from build123d import *

# Parameters (mm, degrees)
F0_R     = 1.55
F0_R_2   = 3
F1_DEPTH = 5
F2_DEPTH = 8


with BuildPart() as f1:
    # F0 (on Top) → F1 (new body)
    with BuildSketch(Plane.XY):
        with BuildLine():
            ThreePointArc((9.1651513899, -4), (9.7890631293, -2.0430964369), (10, 0))
            ThreePointArc((10, 0), (9.7890631293, 2.0430964369), (9.1651513899, 4))
            ThreePointArc((9.1651513899, 4), (5.4772255751, 8.3666002653), (0, 10))
            ThreePointArc((0, 10), (-10, 0), (0, -10))
            ThreePointArc((0, -10), (5.4772255751, -8.3666002653), (9.1651513899, -4))
        make_face()
        with Locations((0, -6.35)):
            Circle(F0_R, mode=Mode.SUBTRACT)
        with Locations((-6.35, 0)):
            Circle(F0_R, mode=Mode.SUBTRACT)
        Circle(F0_R_2, mode=Mode.SUBTRACT)
        with Locations((6.35, 0)):
            Circle(F0_R, mode=Mode.SUBTRACT)
        with Locations((0, 6.35)):
            Circle(F0_R, mode=Mode.SUBTRACT)
        with BuildLine():
            ThreePointArc((0, 10), (5.4772255751, 8.3666002653), (9.1651513899, 4))
            Line((9.1651513899, 4), (90.8348486101, 4))
            ThreePointArc((90.8348486101, 4), (94.5227744249, 8.3666002653), (100, 10))
            Line((100, 10), (0, 10))
        make_face()
        with BuildLine():
            ThreePointArc((100, 10), (94.5227744249, 8.3666002653), (90.8348486101, 4))
            Line((90.8348486101, 4), (100, 4))
            ThreePointArc((100, 4), (102.8284271247, 2.8284271247), (104, 0))
            ThreePointArc((104, 0), (102.8284271247, -2.8284271247), (100, -4))
            Line((100, -4), (90.8348486101, -4))
            ThreePointArc((90.8348486101, -4), (94.5227744249, -8.3666002653), (100, -10))
            ThreePointArc((100, -10), (107.0710678119, -7.0710678119), (110, 0))
            ThreePointArc((110, 0), (107.0710678119, 7.0710678119), (100, 10))
        make_face()
        with BuildLine():
            Line((90.8348486101, -4), (9.1651513899, -4))
            ThreePointArc((9.1651513899, -4), (5.4772255751, -8.3666002653), (0, -10))
            Line((0, -10), (100, -10))
            ThreePointArc((100, -10), (94.5227744249, -8.3666002653), (90.8348486101, -4))
        make_face()
        with BuildLine():
            ThreePointArc((9.1651513899, 4), (9.7890631293, 2.0430964369), (10, 0))
            ThreePointArc((10, 0), (9.7890631293, -2.0430964369), (9.1651513899, -4))
            Line((9.1651513899, -4), (90.8348486101, -4))
            ThreePointArc((90.8348486101, -4), (90, 0), (90.8348486101, 4))
            Line((90.8348486101, 4), (9.1651513899, 4))
        make_face()
        with BuildLine():
            Line((100, 4), (90.8348486101, 4))
            ThreePointArc((90.8348486101, 4), (90, 0), (90.8348486101, -4))
            Line((90.8348486101, -4), (100, -4))
            ThreePointArc((100, -4), (96, 0), (100, 4))
        make_face()
    extrude(amount=F1_DEPTH)

    # F0 (on Top) → F2 (join)
    with BuildSketch(Plane.XY):
        with BuildLine():
            ThreePointArc((9.1651513899, -4), (9.7890631293, -2.0430964369), (10, 0))
            ThreePointArc((10, 0), (9.7890631293, 2.0430964369), (9.1651513899, 4))
            ThreePointArc((9.1651513899, 4), (5.4772255751, 8.3666002653), (0, 10))
            ThreePointArc((0, 10), (-10, 0), (0, -10))
            ThreePointArc((0, -10), (5.4772255751, -8.3666002653), (9.1651513899, -4))
        make_face()
        with Locations((0, -6.35)):
            Circle(F0_R, mode=Mode.SUBTRACT)
        with Locations((-6.35, 0)):
            Circle(F0_R, mode=Mode.SUBTRACT)
        Circle(F0_R_2, mode=Mode.SUBTRACT)
        with Locations((6.35, 0)):
            Circle(F0_R, mode=Mode.SUBTRACT)
        with Locations((0, 6.35)):
            Circle(F0_R, mode=Mode.SUBTRACT)
    extrude(amount=F2_DEPTH)


solid = f1.part
The listing builds one solid part. Answer for the finished solid, in the listing's coordinates (mm). Coordinates: 2 decimals unless noted, no trailing zeros. Loops run counter-clockwise (first coordinate to the right, second up) from the corner with the lowest first, then second, coordinate; pieces in that order, holes last. Notation, with made-up numbers: M 54,-10 L 60,-10 A11 cw 60,3 Z; hole C 11.5,82.25 d1. An arc over 180 degrees is marked long. Answer in a Markdown table with one row per item.
1) Find the intervals of material crossed by probe 1 along X at (y, z) = (-2, 1.75); probe 2 along Y at (x, z) = (100, 3); probe 3 along Z at (x, y) = (66, 1.25), in increasing order.
Answers below:
| item | result |
|---|---|
| probe 1 | -9.8 to -2.24, 2.24 to 96.54, 103.46 to 109.8 |
| probe 2 | -10 to -4, 4 to 10 |
| probe 3 | 0 to 5 |
2) Find section D-D (x = -6.35). Determine the outline of the cut face in (y, z).
Answers below:
| item | result |
|---|---|
| outline | M -7.73,0 L -1.55,0 L -1.55,8 L -7.73,8 Z; M 1.55,0 L 7.73,0 L 7.73,8 L 1.55,8 Z |
3) Determine the mould class of faces 1 (the cylindrical face through (-9.76, 2.17, 4.83)), 2 (the flat face through (54, 0, 5)), 3 (the cylindrical face through (0.715, 4.975, 3.944)) for opening direction X: released by +X, released by -X, zero draft, split by the parting line, or undercut.
Answers below:
| item | result |
|---|---|
| face 1 | split by the parting line |
| face 2 | zero draft |
| face 3 | undercut |
4) Find section C-C (x = 6.35). Determine the outline of the cut face in (y, z), then the cut area to 3 significant figures.
Answers below:
| item | result |
|---|---|
| outline | M -10,0 L -1.55,0 L -1.55,8 L -7.73,8 L -7.73,5 L -10,5 Z; M 1.55,0 L 10,0 L 10,5 L 7.73,5 L 7.73,8 L 1.55,8 Z |
| area | 122 mm^2 |
5) Find section B-B (y = -6.35). Determine the outline of the cut face in (x, z), then the cut area to 3 significant figures.
Answers below:
| item | result |
|---|---|
| outline | M -7.73,0 L -1.55,0 L -1.55,8 L -7.73,8 Z; M 1.55,0 L 107.73,0 L 107.73,5 L 7.73,5 L 7.73,8 L 1.55,8 Z |
| area | 599 mm^2 |
6) Find section A-A (z = 2.25). Determine the outline of the cut face in (x, y).
Answers below:
| item | result |
|---|---|
| outline | M 0,-10 L 100,-10 A10 ccw 100,10 L 0,10 A10 ccw Z; hole C -6.35,0 d3.1; hole C 0,0 d6; hole C 0,-6.35 d3.1; hole C 0,6.35 d3.1; hole C 6.35,0 d3.1; hole C 100,0 d8 |
7) Given pin 1 (5 mm diameter, centred on x = 38, y = -8, fed in from +Z); pin 2 (2.5 mm diameter, centred on x = 0, y = -6.35, fed in from -Z), each flat-ended and moving along its own axis, determine where each tip first touches the part or whether it passes through.
Answers below:
| item | result |
|---|---|
| pin 1 | z = 5 |
| pin 2 | through |
